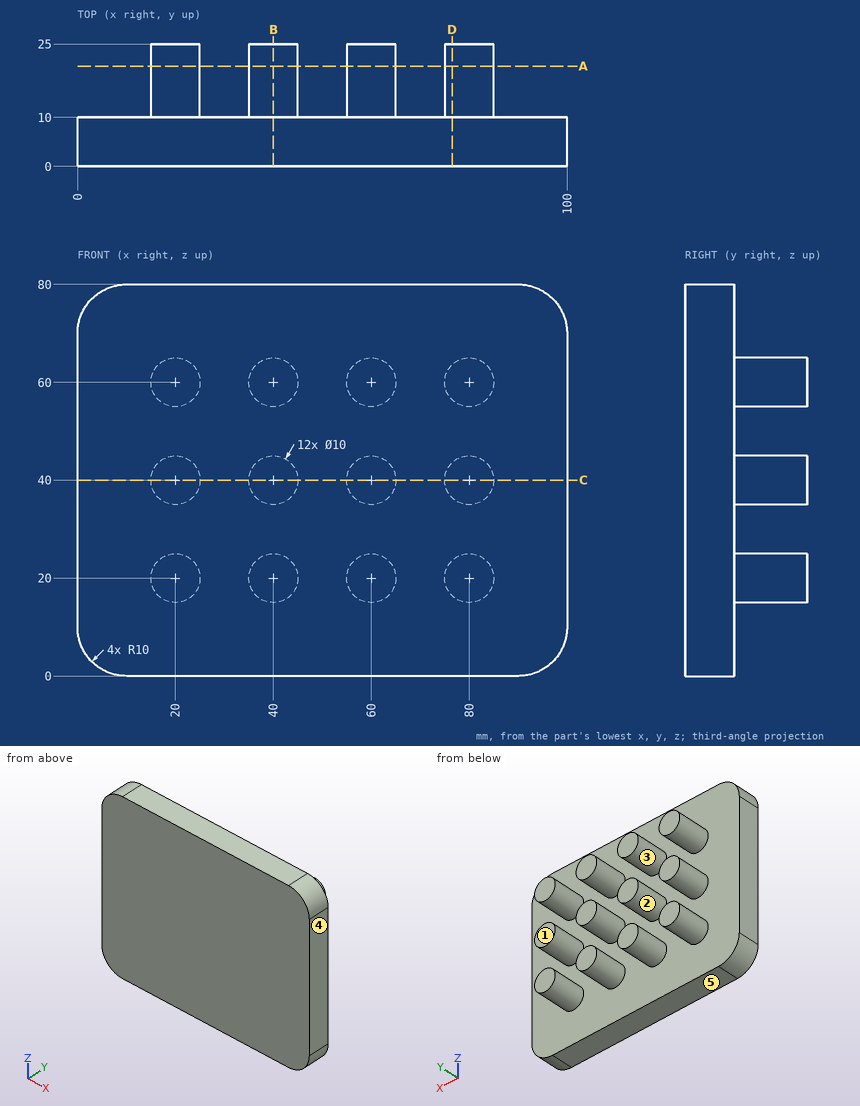
For this review, use the dimensioned drawing (mm, ordinates from the lowest corner) and the shaded views. A direction names the side the tool comes from. Give positions to 0.01 mm unless a question says otherwise; leave off trailing zeros. Write each loop counter-clockwise with the first axis right and the second up, starting at its lowest first coordinate (ties: lowest second). Pieces come first, ordered by that corner, then holes. Notation, with made-up numbers: M 64.5,-32 L 104.5,-32 A17 ccw 104.5,-13 Z; hole C 37.5,52 d9. An arc over 180 degrees is marked long. Write item = value, one per line. Start each with the question number.
Q1. For line 1 (Z direction, x = 38.5, y = 11.5); line 2 (X direction, y = 23.5, z = 16.5); line 3 (X direction, y = 24.25, z = 37), list the stretches that pass through material, from the lowest coordinate up.
Q2. We need section D-D (x = 76.5). State the section outline as (y, z) points.
Q3. We need section C-C (z = 40). State the section outline as (x, y) points.
Q4. Machinability: for the marked faces 1 and 2, which of the approach directions +Z, -Z, +X, -X, +Y, -Y give a long, thin tool a straight path to every point of the face, cutting with its end or side? Answer none if there is none.
Q5. Mouldability with a two-part tool opening along X and no side actions: class the marked faces 3, 4 and 5 as released by +X, released by -X, zero draft, split by the parting line, or undercut.
Q6. We need section B-B (x = 40). State the section outline as (y, z) points, plus the area to 3 significant figures.
Q7. We need section A-A (y = 20.5). Give the number of separate pieces and of enclosed holes in the cut face, plus the area to 3 significant figures.
Q8. Clearance check with flat-ended pins moving along their axes: pin 1 (3 mm diameter, centred on x = 14, z = 51.5, fed in from +Y); pin 2 (12 mm diameter, centred on y = 10.5, z = 52, fed in from +X); pin 3 (5 mm diameter, centred on y = 15, z = 63, fed in from +X). State where each tip first meets the part, or that it passes through.
Result set:
q1.line_1 = 15.23 to 24.77, 35.23 to 44.77, 55.23 to 64.77
q1.line_2 = 16.43 to 23.57, 36.43 to 43.57, 56.43 to 63.57, 76.43 to 83.57
q1.line_3 = 16 to 24, 36 to 44, 56 to 64, 76 to 84
q2.outline = M 0,0 L 10,0 L 10,16.43 L 25,16.43 L 25,23.57 L 10,23.57 L 10,36.43 L 25,36.43 L 25,43.57 L 10,43.57 L 10,56.43 L 25,56.43 L 25,63.57 L 10,63.57 L 10,80 L 0,80 Z
q3.outline = M 0,0 L 100,0 L 100,10 L 85,10 L 85,25 L 75,25 L 75,10 L 65,10 L 65,25 L 55,25 L 55,10 L 45,10 L 45,25 L 35,25 L 35,10 L 25,10 L 25,25 L 15,25 L 15,10 L 0,10 Z
q4.face_1 = +Z, -Z, +X, -X, +Y
q4.face_2 = +Y
q5.face_3 = undercut
q5.face_4 = released by +X
q5.face_5 = zero draft
q6.outline = M 0,0 L 10,0 L 10,15 L 25,15 L 25,25 L 10,25 L 10,35 L 25,35 L 25,45 L 10,45 L 10,55 L 25,55 L 25,65 L 10,65 L 10,80 L 0,80 Z
q6.area = 1,250 mm2
q7.separate_pieces = 12
q7.enclosed_holes = 0
q7.area = 942 mm2
q8.pin_1 = 10
q8.pin_2 = 100
q8.pin_3 = 84.97
